Model file for the job. Use its own axes, mm. Round coordinates to 2 decimals unless told otherwise and drop trailing zeros. Loops run counter-clockwise (first coordinate to the right, second up) from the corner with the lowest first, then second, coordinate; pieces in that order, holes last. Notation, with made-up numbers: (2, -7.5) - (47, -7.5) arc R25 ccw to (47, 13.5) - close; hole circle Ø8 at (86.25, -19.5). An arc over 180 degrees is marked (long way). Answer as a JSON object with one key per item and string values.
from build123d import *

# Parameters (mm, degrees)
F1_DEPTH = 3


with BuildPart() as f1:
    # F0 (on Front) → F1 (new body)
    with BuildSketch(Plane.XZ):
        with BuildLine():
            Line((4.633374, 76.245005), (4.698028, 76.063357))
            Line((4.698028, 76.063357), (4.698028, 29.420612))
            Line((4.698028, 29.420612), (4.698028, 0))
            Line((4.698028, 0), (4.698028, -11.297515))
            Line((4.698028, -11.297515), (48.249803, -11.297515))
            Line((48.249803, -11.297515), (71.0802, -11.297515))
            Line((71.0802, -11.297515), (78.141153, -11.297515))
            Line((78.141153, -11.297515), (78.141153, 0))
            Line((78.141153, 0), (78.151679, 0))
            ThreePointArc((78.151679, 0), (56.35158, 52.389486), (4.859137, 76.231273))
            ThreePointArc((4.859137, 76.231273), (4.74626, 76.238221), (4.633374, 76.245005))
        make_face()
        with BuildLine():
            Line((4.698028, 29.420612), (4.698028, 76.063357))
            Line((4.698028, 76.063357), (4.633374, 76.245005))
            ThreePointArc((4.633374, 76.245005), (2.317706, 76.348073), (0, 76.382439))
            ThreePointArc((0, 76.382439), (-2.317706, 76.348073), (-4.633374, 76.245005))
            Line((-4.633374, 76.245005), (-4.698028, 76.063357))
            Line((-4.698028, 76.063357), (-4.698028, 29.420612))
            Line((-4.698028, 29.420612), (0, 29.420612))
            Line((0, 29.420612), (4.698028, 29.420612))
        make_face()
        with BuildLine():
            Line((4.630308, 76.253618), (4.633374, 76.245005))
            ThreePointArc((4.633374, 76.245005), (4.74626, 76.238221), (4.859137, 76.231273))
            Line((4.859137, 76.231273), (4.855918, 76.239906))
            ThreePointArc((4.855918, 76.239906), (4.743118, 76.246843), (4.630308, 76.253618))
        make_face()
        with BuildLine():
            Line((4.855918, 76.239906), (4.859137, 76.231273))
            ThreePointArc((4.859137, 76.231273), (56.35158, 52.389486), (78.151679, 0))
            Line((78.151679, 0), (78.160097, 0))
            ThreePointArc((78.160097, 0), (56.356415, 52.396601), (4.855918, 76.239906))
        make_face()
        with BuildLine():
            Line((-4.698028, 0), (-4.698028, 29.420612))
            Line((-4.698028, 29.420612), (-4.698028, 76.063357))
            Line((-4.698028, 76.063357), (-4.633374, 76.245005))
            ThreePointArc((-4.633374, 76.245005), (-4.74626, 76.238221), (-4.859137, 76.231273))
            ThreePointArc((-4.859137, 76.231273), (-56.35158, 52.389486), (-78.151679, 0))
            Line((-78.151679, 0), (-78.141153, 0))
            Line((-78.141153, 0), (-78.141153, -11.297515))
            Line((-78.141153, -11.297515), (-71.0802, -11.297515))
            Line((-71.0802, -11.297515), (-48.249803, -11.297515))
            Line((-48.249803, -11.297515), (-4.698028, -11.297515))
            Line((-4.698028, -11.297515), (-4.698028, 0))
        make_face()
        with BuildLine():
            ThreePointArc((-4.859137, 76.231273), (-4.74626, 76.238221), (-4.633374, 76.245005))
            Line((-4.633374, 76.245005), (-4.630308, 76.253618))
            ThreePointArc((-4.630308, 76.253618), (-4.743118, 76.246843), (-4.855918, 76.239906))
            Line((-4.855918, 76.239906), (-4.859137, 76.231273))
        make_face()
        Polygon((71.0802, -11.297515), (48.249803, -11.297515), (56.487575, -35.069365), (64.960711, -35.069365), align=None)
        with BuildLine():
            ThreePointArc((-78.151679, 0), (-56.35158, 52.389486), (-4.859137, 76.231273))
            Line((-4.859137, 76.231273), (-4.855918, 76.239906))
            ThreePointArc((-4.855918, 76.239906), (-56.356415, 52.396601), (-78.160097, 0))
            Line((-78.160097, 0), (-78.151679, 0))
        make_face()
        Polygon((-56.487575, -35.069365), (-48.249803, -11.297515), (-71.0802, -11.297515), (-64.960711, -35.069365), align=None)
    extrude(amount=F1_DEPTH)


solid = f1.part
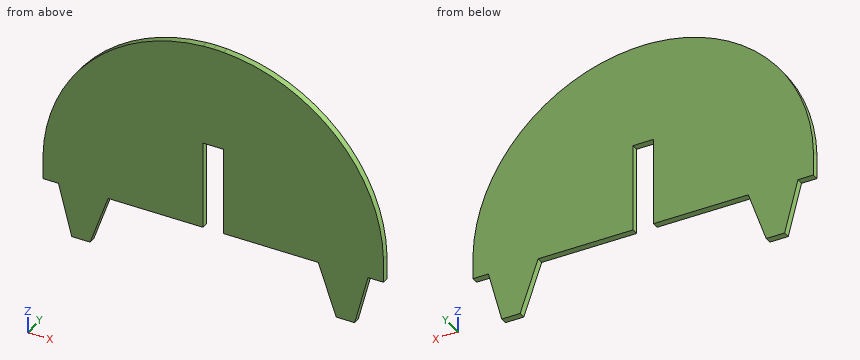
1) Drop flat-ended pins along their axis: P1, Ø1.5, axis at x = 28, y = -1.5, coming from the -Z side; P2, Ø0.9, axis at y = -1.5, z = -6, coming from the +X side; P3, Ø1, axis at y = -1.5, z = 13, coming from the +X side. Give the stop position or say it passes through.
Values follow:
{"P1": "z = -11.3", "P2": "x = 78.14", "P3": "x = 76.86"}
2) Slice it at A-A on y = -0.55. List the corners of the cut face in (x, z) (3 decimals), then the cut area to 3 significant figures.
Values follow:
{"outline": "(-78.16, 0) - (-78.141, 0) - (-78.141, -11.298) - (-71.08, -11.298) - (-64.961, -35.069) - (-56.488, -35.069) - (-48.25, -11.298) - (-4.698, -11.298) - (-4.698, 29.421) - (4.698, 29.421) - (4.698, -11.298) - (48.25, -11.298) - (56.488, -35.069) - (64.961, -35.069) - (71.08, -11.298) - (78.141, -11.298) - (78.141, 0) - (78.16, 0) arc R78.181 ccw to (4.856, 76.24) arc R78.69 ccw to (4.63, 76.254) - (4.633, 76.245) arc R78.172 ccw to (0, 76.382) arc R78.172 ccw to (-4.633, 76.245) - (-4.63, 76.254) arc R78.69 ccw to (-4.856, 76.24) arc R78.181 ccw to start", "area": "11,400 mm²"}
3) Slice it at C-C on z = 12. List the corners of the cut face in (x, y).
Values follow:
{"outline": "(-76.95, -3) - (-4.7, -3) - (-4.7, 0) - (-76.95, 0) - close; (4.7, -3) - (76.95, -3) - (76.95, 0) - (4.7, 0) - close"}
4) Slice it at B-B on z = -25. List the corners of the cut face in (x, y), then the cut area to 3 significant figures.
Values follow:
{"outline": "(-67.55, -3) - (-53, -3) - (-53, 0) - (-67.55, 0) - close; (53, -3) - (67.55, -3) - (67.55, 0) - (53, 0) - close", "area": "87.3 mm²"}
5) Probe probe 1 along X at (y, z) = (-0.3, -7.5); probe 2 along Z at (x, y) = (1, -1.1); probe 3 along X at (y, z) = (-2.7, -18). List the from-to ranges inside material, lowest first.
Values follow:
{"probe 1": "-78.14 to -4.7, 4.7 to 78.14", "probe 2": "29.42 to 76.38", "probe 3": "-69.35 to -50.57, 50.57 to 69.35"}
6) Slice it at D-D on x = 29. List the corners of the cut face in (y, z).
Values follow:
{"outline": "(-3, -11.3) - (0, -11.3) - (0, 70.81) - (-3, 70.81) - close"}
